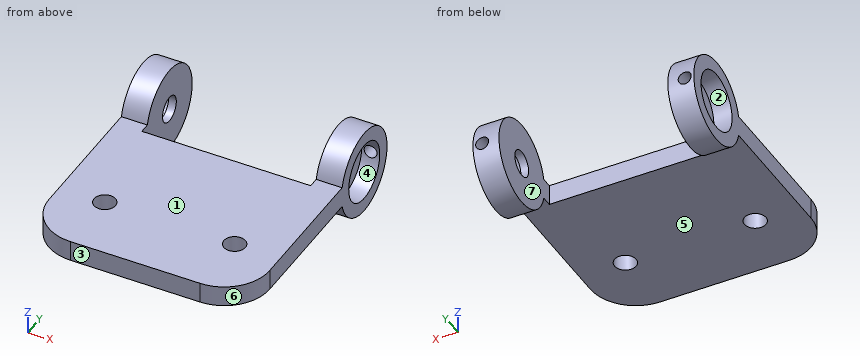
```python
from build123d import *

# Parameters (mm, degrees)
BOSS_EXTRUDE1_DEPTH = 4
SKETCH7_R           = 4.15
BOSS_EXTRUDE3_DEPTH = 8
SKETCH8_R           = 16.5
BOSS_EXTRUDE4_DEPTH = 10
SKETCH9_R           = 11.25
CUT_EXTRUDE1_DEPTH  = 7
SKETCH10_R          = 5
CUT_EXTRUDE2_DEPTH  = 3
SKETCH11_R          = 2.5
CUT_EXTRUDE3_DEPTH  = 10


with BuildPart() as part:
    # Sketch2 → Boss-Extrude1 (new, symmetric)
    with BuildSketch(Plane.XY):
        Polygon((-42.5, 13.75), (-32.5, 13.75), (-32.5, -13.75), (32.5, -13.75), (32.5, 13.75), (42.5, 13.75), (42.5, -23.75), (-42.5, -23.75), align=None)
    extrude(amount=BOSS_EXTRUDE1_DEPTH, both=True)

    # Sketch7 → Boss-Extrude3 (add)
    with BuildSketch(Plane.XY.offset(4)):
        with BuildLine():
            Line((-42.5, -23.75), (-42.5, -62.25))
            ThreePointArc((-42.5, -62.25), (-37.374368671, -74.624368671), (-25, -79.75))
            Line((-25, -79.75), (25, -79.75))
            ThreePointArc((25, -79.75), (37.374368671, -74.624368671), (42.5, -62.25))
            Line((42.5, -62.25), (42.5, -23.75))
            Line((42.5, -23.75), (-42.5, -23.75))
        make_face()
        with Locations((-25, -54.75)):
            Circle(SKETCH7_R, mode=Mode.SUBTRACT)
        with Locations((25, -54.75)):
            Circle(SKETCH7_R, mode=Mode.SUBTRACT)
    extrude(amount=-BOSS_EXTRUDE3_DEPTH)

    # Sketch8 → Boss-Extrude4 (add)
    with BuildSketch(Plane.ZY.offset(42.5)):
        with Locations((0, 6.25)):
            Circle(SKETCH8_R)
    boss_extrude4 = extrude(amount=-BOSS_EXTRUDE4_DEPTH)

    # Sketch9 → Cut-Extrude1 (cut)
    with BuildSketch(Plane.ZY.offset(42.5)):
        with Locations((0, 6.25)):
            Circle(SKETCH9_R)
    cut_extrude1 = extrude(amount=-CUT_EXTRUDE1_DEPTH, mode=Mode.SUBTRACT)

    # Sketch10 → Cut-Extrude2 (cut)
    with BuildSketch(Plane.ZY.offset(35.5)):
        with Locations((0, 6.25)):
            Circle(SKETCH10_R)
    cut_extrude2 = extrude(amount=-CUT_EXTRUDE2_DEPTH, mode=Mode.SUBTRACT)

    # Mirror1: Boss-Extrude4, Cut-Extrude1, Cut-Extrude2 across plane
    add(boss_extrude4.mirror(Plane(origin=(0, 0, 0), x_dir=(0, 0, 1), z_dir=(1, 0, 0))))
    add(cut_extrude1.mirror(Plane(origin=(0, 0, 0), x_dir=(0, 0, 1), z_dir=(1, 0, 0))), mode=Mode.SUBTRACT)
    add(cut_extrude2.mirror(Plane(origin=(0, 0, 0), x_dir=(0, 0, 1), z_dir=(1, 0, 0))), mode=Mode.SUBTRACT)

    # Sketch11 → Cut-Extrude3 (cut)
    with BuildSketch(Plane(origin=(0, 22.75, 0), x_dir=(1, 0, 0), z_dir=(0, 1, 0))):
        with Locations(Location((-39, 0, 0), (0, 0, 270))):
            Circle(SKETCH11_R)
        with Locations(Location((39, 0, 0), (0, 0, 270))):
            Circle(SKETCH11_R)
    extrude(amount=-CUT_EXTRUDE3_DEPTH, mode=Mode.SUBTRACT)


solid = part.part
```
Verification items for the finished model (mm, model axes). Face numbers are marked on the shaded views. A direction names the side the tool comes from. Give positions to 0.01 mm unless a question says otherwise; leave off trailing zeros. Order: outer loops, then holes, each group sorted by start corner. A loop starts at its lowest first (then second) coordinate and runs counter-clockwise, first axis right, second up. Notation, with made-up numbers: (27.5, -34) -> (86.5, -34) arc R4 ccw to (86.5, -29) -> close; hole circle Ø9 at (-17, 18.5). An arc over 180 degrees is marked (long way). One line per item, written item: value.
(1) Sectioned sample at C-C on z = 7. Record the cut outline in (x, y), then the cut area to 3 significant figures.
Final values:
outline: (-42.5, -8.69) -> (-32.5, -8.69) -> (-32.5, 21.19) -> (-42.5, 21.19) -> (-42.5, 15.06) -> (-35.5, 15.06) -> (-35.5, -2.56) -> (-42.5, -2.56) -> close; (32.5, -8.69) -> (42.5, -8.69) -> (42.5, -2.56) -> (35.5, -2.56) -> (35.5, 15.06) -> (42.5, 15.06) -> (42.5, 21.19) -> (32.5, 21.19) -> close
area: 351 mm^2
(2) Sectioned sample at B-B on y = 6.25. Record the cut outline in (x, z).
Final values:
outline: (-42.5, -16.5) -> (-32.5, -16.5) -> (-32.5, -5) -> (-35.5, -5) -> (-35.5, -11.25) -> (-42.5, -11.25) -> close; (-42.5, 11.25) -> (-35.5, 11.25) -> (-35.5, 5) -> (-32.5, 5) -> (-32.5, 16.5) -> (-42.5, 16.5) -> close; (32.5, -16.5) -> (42.5, -16.5) -> (42.5, -11.25) -> (35.5, -11.25) -> (35.5, -5) -> (32.5, -5) -> close; (32.5, 5) -> (35.5, 5) -> (35.5, 11.25) -> (42.5, 11.25) -> (42.5, 16.5) -> (32.5, 16.5) -> close
(3) Draft check along Y on the marked faces 1, 2, 3 and 4. Enter one of: pulls with the +Y half, pulls with the -Y half, needs draft (parallel to the pull), parting line crosses it, or undercut.
Final values:
face 1: needs draft
face 2: undercut
face 3: pulls with the -Y half
face 4: undercut
(4) Sectioned sample at D-D on x = -27. Record the cut outline in (y, z).
Final values:
outline: (-79.64, -4) -> (-58.39, -4) -> (-58.39, 4) -> (-79.64, 4) -> close; (-51.11, -4) -> (-13.75, -4) -> (-13.75, 4) -> (-51.11, 4) -> close
(5) Tool access check on the marked faces 5, 6 and 7. Record the directions out of +Z, -Z, +X, -X, +Y, -Y that give a thin tool (end or side, any length) a straight path to the whole face; none if there is none.
Final values:
face 5: -Z, +X, -X, -Y
face 6: +Z, -Z, +X, -Y
face 7: +Z, -Z, +Y
(6) Sectioned sample at A-A on y = -54.75. Record the cut outline in (x, z).
Final values:
outline: (-42.5, -4) -> (-29.15, -4) -> (-29.15, 4) -> (-42.5, 4) -> close; (-20.85, -4) -> (20.85, -4) -> (20.85, 4) -> (-20.85, 4) -> close; (29.15, -4) -> (42.5, -4) -> (42.5, 4) -> (29.15, 4) -> close
(7) Scan lines: line 1 along X through (y, z) = (19.25, 0); line 2 along Z through (x, y) = (-34, 6); line 3 along Y through (x, z) = (-25, 1). Record each from-to range of solid material in increasing order. Write a range as [from, to].
Final values:
line 1: [-42.5, -41.5], [-36.5, -32.5], [32.5, 36.5], [41.5, 42.5]
line 2: [-16.5, -4.99], [4.99, 16.5]
line 3: [-79.75, -58.9], [-50.6, -13.75]
(8) Gauge pin test, flat ends, axial feed: pin 1 (11.5 mm diameter, centred on y = 6.25, z = 0, fed in from +X); pin 2 (6.5 mm diameter, centred on x = 14, z = 1.5, fed in from +Y); pin 3 (5 mm diameter, centred on x = 25, y = -54.75, fed in from -Z); pin 4 (11.5 mm diameter, centred on y = 6.25, z = 0, fed in from -X). Record the tip position at first contact, or that the pin passes through.
Final values:
pin 1: x = 35.5
pin 2: y = -13.75
pin 3: through
pin 4: x = -35.5
